Input: part model. Units: mm. Frame: model coordinates. Face numbers are marked on the shaded views. A direction names the side the tool comes from. Give positions to 0.01 mm unless a question says otherwise; leave off trailing zeros. Loops run counter-clockwise (first coordinate to the right, second up) from the corner with the lowest first, then second, coordinate; pieces in that order, holes last. Notation, with made-up numbers: (74, 26) - (106, 26) arc R25 ccw to (106, 42) - close; hole circle Ø1 at (5, -14.5). An arc over 180 degrees is marked (long way). Answer as a JSON object with one key per item and string values. Group by question number.
(1) Material intervals for L1, parallel to Z at x = 3.5, y = 0; L2, parallel to X at y = 0.25, z = -9.75; L3, parallel to X at y = 2.75, z = 3, sorted ascending.
(2) Section query B-B (z = -7.5). Return loops of the section in (x, y), plus the area to 3 significant figures.
(3) Access query for the marked faces 1 and 2. Directions: +Z, -Z, +X, -X, +Y, -Y. A direction counts if a zero-diameter tool reaches every point of the face in a straight line with its end or side. Return the directions, or none.
(4) Section query A-A (y = 0). Return loops of the section in (x, z), plus the area to 3 significant figures.
(5) Section query D-D (y = 2.75). Return loops of the section in (x, z).
(6) Section query C-C (y = -3.75). Return loops of the section in (x, z), plus the area to 3 significant figures.
(7) Pin query (flat end, axial travel): P1, Ø3, axis at y = 2.5, z = -6.5, coming from the +X side. Return the tip coordinate at first contact, or that it passes through.
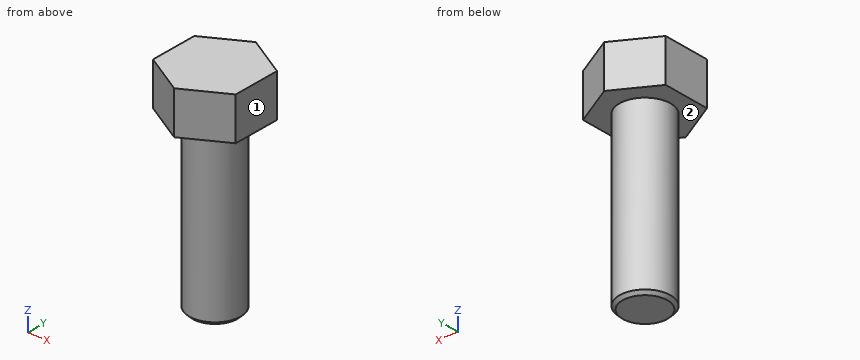
Autodesk Inventor part; units mm, degrees
ref_plane "YZ Plane" through (0, 0, 0) normal (1, 0, 0) x (0, 1, 0)
ref_plane "XZ Plane" through (0, 0, 0) normal (0, 1, 0) x (-1, 0, 0)
ref_plane "XY Plane" through (0, 0, 0) normal (0, 0, 1) x (1, 0, 0)
sketch "Эскиз1" plane through (0, 0, 0) normal (0, 0, 1) x (1, 0, 0)
  line L0 (0, -4.45) -> (-3.9, -2.2517)
  line L1 (3.9, -2.2517) -> (0, -4.45)
  line L2 (0, 4.45) -> (3.9, 2.2517)
  line L3 (-3.9, 2.2517) -> (0, 4.45)
  line L4 (-3.9, -2.2517) -> (-3.9, 2.2517)
  line L5 (3.9, -2.2517) -> (3.9, 2.2517)
  point P0 (0, 0)
extrude "Выдавливание1" add sketch "Эскиз1" along normal blind 4
sketch "Эскиз2" plane through (0, 0, 0) normal (0, 0, -1) x (-1, 0, 0)
  circle A0 centre (0, 0) radius 2.4
  dimension "d2" = 4.8
extrude "Выдавливание2" add sketch "Эскиз2" along normal blind 16
thread "Резьба1"
chamfer "Фаска1" distance 0.3 angle 45 1 edges at (2.4, 0, -16)
properties part number "Болт М5х16"
Recorded:
{
 "1": {"L1": "z = 0 to 4", "L2": "x = -2.39 to 2.39", "L3": "x = -3.02 to 3.02"},
 "2": {"outline": "circle Ø4.8 at (0, 0)", "area": "18.1 mm^2"},
 "3": {"face 1": "+Z, -Z, +X, +Y, -Y", "face 2": "-Z"},
 "4": {"outline": "(-3.9, 0) - (-2.4, 0) - (-2.4, -15.7) - (-2.1, -16) - (2.1, -16) - (2.4, -15.7) - (2.4, 0) - (3.9, 0) - (3.9, 4) - (-3.9, 4) - close", "area": "108 mm^2"},
 "5": {"outline": "(-3.02, 0) - (3.02, 0) - (3.02, 4) - (-3.02, 4) - close"},
 "6": {"outline": "(-1.24, 0) - (1.24, 0) - (1.24, 4) - (-1.24, 4) - close", "area": "9.93 mm^2"},
 "7": {"P1": "stops at x = 2.18"}
}
